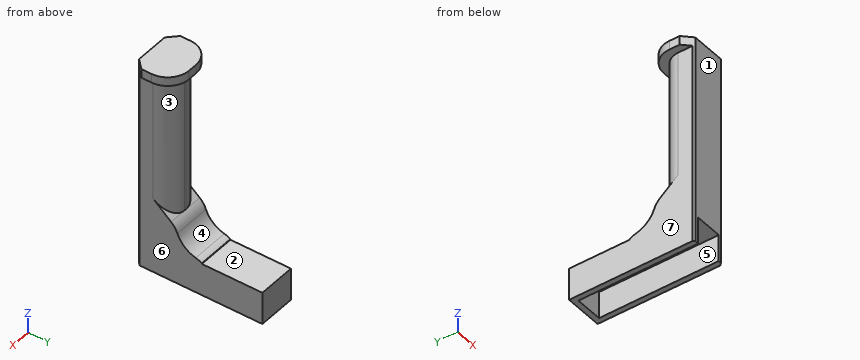
```python
from build123d import *

# Parameters (mm, degrees)
SKETCH1_W           = 21.3
SKETCH1_H           = 70
BOSS_EXTRUDE1_DEPTH = 3
BOSS_EXTRUDE2_DEPTH = 15.1
SKETCH3_W           = 15.400000000000002
SKETCH3_H           = 3
BOSS_EXTRUDE3_DEPTH = 15.1
BOSS_EXTRUDE4_DEPTH = 95
BOSS_EXTRUDE5_DEPTH = 5
SKETCH9_W           = 21.3
SKETCH9_H           = 17.22200087142766
BOSS_EXTRUDE6_DEPTH = 16.000000000000007
SKETCH12_R          = 14.60799399049553
CUT_EXTRUDE1_DEPTH  = 109.85245207766768
CHAMFER4_SIZE       = 1
CHAMFER5_SIZE       = 5
CHAMFER6_SIZE       = 5
FILLET4_R           = 12
FILLET5_R           = 12
FILLET6_R           = 12
FILLET7_R           = 10


with BuildPart() as part:
    # Sketch1 → Boss-Extrude1 (new body)
    with BuildSketch(Plane.XY):
        Rectangle(SKETCH1_W, SKETCH1_H)
    extrude(amount=-BOSS_EXTRUDE1_DEPTH)

    # Sketch2 → Boss-Extrude2 (add)
    with BuildSketch(Plane(origin=(0, 0, -3), x_dir=(-1, 0, 0), z_dir=(0, 0, -1))):
        Polygon((-10.649999999999999, 35), (-7.700000000000009, 35), (-7.700000000000002, -35), (-10.649999999999999, -35), align=None)
        Polygon((10.650000000000002, 35), (7.699999999999991, 35), (7.699999999999998, -35), (10.650000000000002, -35), align=None)
    extrude(amount=BOSS_EXTRUDE2_DEPTH)

    # Sketch3 → Boss-Extrude3 (add)
    with BuildSketch(Plane(origin=(0, 0, -3), x_dir=(-1, 0, 0), z_dir=(0, 0, -1))):
        with Locations((-9.33e-15, 33.5)):
            Rectangle(SKETCH3_W, SKETCH3_H)
    extrude(amount=BOSS_EXTRUDE3_DEPTH)

    # Sketch4 → Boss-Extrude4 (add)
    with BuildSketch(Plane.XY):
        Polygon((-10.650000000000002, -16.099065593181194), (10.649999999999999, -16.099065593181194), (10.650000000000007, -35), (-10.649999999999993, -35), align=None)
    extrude(amount=BOSS_EXTRUDE4_DEPTH)

    # Sketch6 → Boss-Extrude5 (add)
    with BuildSketch(Plane.XY.offset(95)):
        Polygon((-14.790899735714902, -12.21473987671473), (14.327115992863071, -12.21473987671473), (14.327115992863074, -35), (-14.790899735714893, -35), align=None)
    extrude(amount=BOSS_EXTRUDE5_DEPTH)

    # Sketch9 → Boss-Extrude6 (add)
    with BuildSketch(Plane.XY):
        with Locations((-1.78e-15, -7.488065157467364)):
            Rectangle(SKETCH9_W, SKETCH9_H)
    extrude(amount=BOSS_EXTRUDE6_DEPTH)

    # Sketch12 → Cut-Extrude1 (cut, through all)
    with BuildSketch(Plane.ZY.offset(10.650000000000002)):
        with Locations((16.000000000000007, 1.122935278246466)):
            Circle(SKETCH12_R)
    extrude(amount=-CUT_EXTRUDE1_DEPTH, mode=Mode.SUBTRACT)

    # Chamfer3
    # the kernel refuses this chamfer: 3 mm, written as the material it takes off along each edge
    with BuildSketch(Plane(origin=(17.73850714382705, -13.485058712249064, 16.000000000000007), x_dir=(0, 0.08550168468531993, -0.9963380259309449), z_dir=(-1, 0, 0))) as chamfer3_piece_1_section:
        with BuildLine():
            Line((2.582869005863168, -0.08485281374238583), (-0.31934564535848514, 2.817361837479259))
            Line((-0.31934564535848514, 2.817361837479259), (-0.37912592691434055, 2.81223173639814))
            ThreePointArc((-0.37912592691434055, 2.81223173639814), (-0.18095110257164257, 1.4068549031398474), (-0.05978028155585542, -0.00513010108111909))
            Line((-0.05978028155585542, -0.00513010108111909), (0.00513010108111924, -0.05978028155585719))
            ThreePointArc((0.00513010108111924, -0.05978028155585719), (1.2915393356537215, -0.00656807524010173), (2.5777389047820485, -0.1446330952982423))
            Line((2.5777389047820485, -0.1446330952982423), (2.582869005863168, -0.08485281374238583))
        make_face()
    chamfer3_piece_1 = extrude(amount=35.4770142876541, mode=Mode.PRIVATE)
    chamfer3_piece_1 = split(chamfer3_piece_1, bisect_by=Plane(origin=(17.73850714382705, -16.099065593181194, 16.000000000000007), z_dir=(0, 1, 0)), keep=Keep.TOP, mode=Mode.PRIVATE)
    add(chamfer3_piece_1, mode=Mode.SUBTRACT)

    # Chamfer4
    # the kernel refuses this chamfer: 1 mm, written as the material it takes off along each edge
    with BuildSketch(Plane(origin=(13.31779092299838, 1.122935278246466, 1.3920060095044775), x_dir=(0, -0.9993692754635791, 0.0355112835504551), z_dir=(-1, 0, 0))) as chamfer4_piece_1:
        with BuildLine():
            Line((1.0374972333996406, 1e-17), (-CHAMFER4_SIZE * 0.0355112835505, -CHAMFER4_SIZE * 0.999369275464))
            Line((-CHAMFER4_SIZE * 0.0355112835505, -CHAMFER4_SIZE * 0.999369275464), (0, 0))
            ThreePointArc((0, 0), (0.5334069539111667, -0.00920626580887721), (1.0374972333996406, 1e-17))
        make_face()
    extrude(amount=26.63558184599676, mode=Mode.SUBTRACT)

    # Chamfer5
    chamfer5_edges = [part.edges().sort_by_distance(p)[0] for p in [
        (-14.790899735714893, -35, 97.5),
    ]]
    chamfer(chamfer5_edges, length=CHAMFER5_SIZE)

    # Chamfer6
    chamfer6_edges = [part.edges().sort_by_distance(p)[0] for p in [
        (14.327115992863074, -35, 97.5),
    ]]
    chamfer(chamfer6_edges, length=CHAMFER6_SIZE)

    # Fillet4
    fillet4_edges = [part.edges().sort_by_distance(p)[0] for p in [
        (14.327115992863071, -12.21473987671473, 97.5),
        (-14.790899735714902, -12.21473987671473, 97.5),
    ]]
    fillet(fillet4_edges, radius=FILLET4_R)

    # Fillet5
    fillet5_edges = [part.edges().sort_by_distance(p)[0] for p in [
        (-1.78e-15, -13.271474119451348, 13.511131478397797),
    ]]
    fillet(fillet5_edges, radius=FILLET5_R)

    # Fillet6
    # the kernel refuses this fillet: 12 mm, written as the material it takes off along each edge
    with BuildSketch(Plane(origin=(16.66324146618684, 0.086092419807557, 1.428848867941594), x_dir=(0, -0.9882482751789802, 0.15285727527916634), z_dir=(-1, 0, 0))) as fillet6_piece_1:
        with BuildLine():
            CenterArc((3.393233706942116, -11.959263365525597), FILLET6_R, 94.7223972339899, 17.695866700852164)
            Line((-1.1831471407174274, -0.8661691922493711), (-1.274674757670618, -0.6443073087838466))
            ThreePointArc((-1.274674757670618, -0.6443073087838466), (-0.7333441241917547, -0.2394325626577685), (-0.1417705538330419, 0.19365203346691875))
            Line((-0.1417705538330419, 0.19365203346691875), (0.01975874240954748, 0.23918526731049536))
            ThreePointArc((0.01975874240954748, 0.23918526731049536), (1.2026482932374447, 0.19040995736707406), (2.38553784406539, 0.23918526731051196))
            Line((2.38553784406539, 0.23918526731051196), (2.405296586474737, 0))
        make_face()
    extrude(amount=33.32648293237368, mode=Mode.SUBTRACT)

    # Fillet7
    fillet7_edges = [part.edges().sort_by_distance(p)[0] for p in [
        (-10.650000000000002, -16.099065593181095, 55.44588674849325),
        (10.649999999999999, -16.099065593181095, 55.44588674849325),
    ]]
    fillet(fillet7_edges, radius=FILLET7_R)


solid = part.part
```
Geometry check sheet. Reference: the model listing, model coordinates, mm. Face numbers are marked on the shaded views. A direction names the side the tool comes from. Coordinates: 2 decimals unless noted, no trailing zeros. Order: outer loops, then holes, each group sorted by start corner. A loop starts at its lowest first (then second) coordinate and runs counter-clockwise, first axis right, second up. Notation, with made-up numbers: M 37.25,87.25 L 58.25,87.25 A10 ccw 58.25,104.25 Z; hole C -22.5,2 d11. An arc over 180 degrees is marked long. One line per question, with ' | ' between items. Start each with the question number.
Item 1: Draft check along X on the marked faces 4, 5, 6 and 7. Enter one of: pulls with the +X half, pulls with the -X half, needs draft (parallel to the pull), parting line crosses it, or undercut.
Item 2: Cross-section at D-D on z = -4.5. Enter the section's corners in (x, y), then the cut area to 3 significant figures.
Item 3: Cross-section at C-C on x = 5.5. Enter the section's corners in (y, z), then the cut area to 3 significant figures.
Item 4: Cross-section at B-B on y = 12. Enter the section's corners in (x, z).
Item 5: Material ranges on L1, parallel to X at y = 29.5, z = -7.5; L2, parallel to Z at x = -7.5, y = 18; L3, parallel to Z at x = -1, y = -21.5, recorded low to high. Write a range as [from, to].
Item 6: Set-up check for the marked faces 1, 2 and 3: record each of +Z, -Z, +X, -X, +Y, -Y from which the full face is reachable in a straight line by a thin tool's end or side.
Item 7: Gauge pin test, flat ends, axial feed: pin 1 (4.5 mm diameter, centred on x = 1, z = -12, fed in from -Y); pin 2 (1 mm diameter, centred on x = 10.5, z = 74, fed in from -Y); pin 3 (4 mm diameter, centred on x = 2, y = -15.5, fed in from -Z). Record the tip position at first contact, or that the pin passes through.
Item 8: Cross-section at A-A on z = 49. Enter the section's corners in (x, y).
Findings:
1) face 4: needs draft | face 5: undercut | face 6: pulls with the +X half | face 7: pulls with the -X half
2) outline: M -10.65,-34.14 L -9.79,-35 L -7.7,-35 L -7.7,32 L 7.7,32 L 7.7,-35 L 9.33,-35 L 10.65,-33.68 L 10.65,35 L -10.65,35 Z | area: 458 mm²
3) outline: M -35,-3 L 32,-3 L 32,-18.1 L 35,-18.1 L 35,0 L 1.12,0 L 1.12,0.39 A12 ccw -2.29,1.8 A14.61 cw -12.56,10.89 A12 ccw -16.08,15.87 L -17.35,16.95 L -17.35,95 L -12.64,95 L -12.64,100 L -35,100 Z | area: 2,170 mm²
4) outline: M -10.65,-18.1 L -7.7,-18.1 L -7.7,-3 L 7.7,-3 L 7.7,-18.1 L 10.65,-18.1 L 10.65,0 L -10.65,0 Z
5) L1: x = [-10.65, -7.7], [7.7, 10.65] | L2: z = [-3, 0] | L3: z = [-3, 100]
6) face 1: +Z, -Z, +X, -X, -Y | face 2: +Z, +X, -X, +Y | face 3: +X, +Y
7) pin 1: stops at y = 32 | pin 2: stops at y = -34.33 | pin 3: stops at z = -3
8) outline: M -10.65,-34.14 L -9.79,-35 L 9.33,-35 L 10.65,-33.68 L 10.65,-26.1 A10 ccw 0.65,-16.1 L -0.65,-16.1 A10 ccw -10.65,-26.1 Z
